```python
from build123d import *

# Parameters (mm, degrees)
T_LE_DE_BASE_PLI_E1_DEPTH = 35
ESQUISSE14_R              = 1.5
ENL_V_MAT_EXTRU_1_DEPTH   = 2
ESQUISSE15_R              = 3.5
ESQUISSE15_R_2            = 1.5
ENL_V_MAT_EXTRU_2_DEPTH   = 2


# Sheet-metal steps are written as plain solids
with BuildPart() as part:
    # Esquisse8 → Tôle de base pliée1 (new body)
    with BuildSketch(Plane.XY):
        with BuildLine():
            Line((-35, 0), (-0.7366, 0))
            ThreePointArc((-0.7366, 0), (-0.215745145, -0.215745145), (0, -0.7366))
            Line((0, -0.7366), (0, -45))
            Line((0, -45), (2, -45))
            Line((2, -45), (2, -0.7366))
            ThreePointArc((2, -0.7366), (1.198468417, 1.198468417), (-0.7366, 2))
            Line((-0.7366, 2), (-35, 2))
            Line((-35, 2), (-35, 0))
        make_face()
    extrude(amount=T_LE_DE_BASE_PLI_E1_DEPTH)

    # Esquisse14 → Enlèv. mat.-Extru.1 (cut)
    with BuildSketch(Plane(origin=(0, 2, 0), x_dir=(1, 0, 0), z_dir=(0, 1, 0))):
        with Locations(Location((-27, -7, 0), (0, 0, 270))):
            Circle(ESQUISSE14_R)
        with Locations(Location((-8.7366, -7, 0), (0, 0, 270))):
            Circle(ESQUISSE14_R)
        with Locations(Location((-8.7366, -28, 0), (0, 0, 270))):
            Circle(ESQUISSE14_R)
        with Locations(Location((-27, -28, 0), (0, 0, 270))):
            Circle(ESQUISSE14_R)
    extrude(amount=-ENL_V_MAT_EXTRU_1_DEPTH, mode=Mode.SUBTRACT)

    # Esquisse15 → Enlèv. mat.-Extru.2 (cut)
    with BuildSketch(Plane(origin=(2, 0, 0), x_dir=(0, 0, -1), z_dir=(1, 0, 0))):
        with Locations(Location((-17.5, -37, 0), (0, 0, 90))):
            Circle(ESQUISSE15_R)
        with Locations(Location((-9, -37, 0), (0, 0, 90))):
            Circle(ESQUISSE15_R_2)
        with Locations(Location((-26, -37, 0), (0, 0, 90))):
            Circle(ESQUISSE15_R_2)
    extrude(amount=-ENL_V_MAT_EXTRU_2_DEPTH, mode=Mode.SUBTRACT)


solid = part.part
```
Could you check a few things on this model? Use its own coordinates, in mm. A direction names the side the tool comes from. Give positions to 0.01 mm unless a question says otherwise; leave off trailing zeros. Loops run counter-clockwise (first coordinate to the right, second up) from the corner with the lowest first, then second, coordinate; pieces in that order, holes last. Notation, with made-up numbers: (-40, 31.25) - (19, 31.25) arc R25 ccw to (19, 49.25) - close; hole circle Ø5 at (71, -36). An arc over 180 degrees is marked (long way). Answer in a Markdown table with one row per item. Add a question column.
Q1. If we section it at D-D (y = -8): List the corners of the cut face in (x, z) for me, plus the area to 3 significant figures.
Q2. Which directions (+Z, -Z, +X, -X, +Y, -Y) give clear straight access to the entire face, cutting with the end or side of a thin tool? Please do faces 4 (the face through (0, -23, 17)), 5 (the face through (-25.513, 1.014, 6.805)).
Q3. We'd pull the mould along X, two halves only. Please class faces 1 (the face through (-18, 2, 17)), 2 (the face through (-10.2, 1.01, 6.67)), 3 (the face through (-35, 1, 17)): +X half, -X half, draft (parallel to the pull), parting line (faces both ways), or undercut.
Q4. If we section it at C-C (z = 17.5): List the corners of the cut face in (x, y) for me.
Q5. If we section it at B-B (x = -27): List the corners of the cut face in (y, z) for me.
Q6. For pin 1 (4 mm diameter, centred on y = -37, z = 26, fed in from -X); pin 2 (1.8 mm diameter, centred on x = -8.74, z = 28, fed in from +Y); pin 3 (4 mm diameter, centred on x = -27, z = 28, fed in from -Y), each with a flat end and sliding along its axis, tell me the tip position at first contact or that it passes through.
Q7. Please list where these lines run through material, in increasing order: L1, parallel to Z at x = 1.2, y = -37; L2, parallel to X at y = 1.35, z = 28; L3, parallel to X at y = -15.5, z = 15. Write a range as from..to.
Q8. If we section it at A-A (y = -37): List the corners of the cut face in (x, z) for me, plus the area to 3 significant figures.
The answers:
| question | item | result |
|---|---|---|
| 1 | outline | (0, 0) - (2, 0) - (2, 35) - (0, 35) - close |
| 1 | area | 70.0 mm^2 |
| 2 | face 4 | +Z, -Z, -X, -Y |
| 2 | face 5 | +Y, -Y |
| 3 | face 1 | draft |
| 3 | face 2 | undercut |
| 3 | face 3 | -X half |
| 4 | outline | (-35, 0) - (-0.74, 0) arc R0.74 cw to (0, -0.74) - (0, -33.5) - (2, -33.5) - (2, -0.74) arc R2.74 ccw to (-0.74, 2) - (-35, 2) - close; (0, -45) - (2, -45) - (2, -40.5) - (0, -40.5) - close |
| 5 | outline | (0, 0) - (2, 0) - (2, 5.5) - (0, 5.5) - close; (0, 8.5) - (2, 8.5) - (2, 26.5) - (0, 26.5) - close; (0, 29.5) - (2, 29.5) - (2, 35) - (0, 35) - close |
| 6 | pin 1 | stops at x = 0 |
| 6 | pin 2 | passes through |
| 6 | pin 3 | stops at y = 0 |
| 7 | L1 | z = 0..7.5, 10.5..14, 21..24.5, 27.5..35 |
| 7 | L2 | x = -35..-28.5, -25.5..-10.24, -7.24..1.03 |
| 7 | L3 | x = 0..2 |
| 8 | outline | (0, 0) - (2, 0) - (2, 7.5) - (0, 7.5) - close; (0, 10.5) - (2, 10.5) - (2, 14) - (0, 14) - close; (0, 21) - (2, 21) - (2, 24.5) - (0, 24.5) - close; (0, 27.5) - (2, 27.5) - (2, 35) - (0, 35) - close |
| 8 | area | 44.0 mm^2 |
